from build123d import *

# Parameters (mm, degrees)
F0_R     = 1.55
F1_DEPTH = 3
F3_DEPTH = 3
F4_R     = 1.25
F5_DEPTH = 3
F6_SIZE  = 0.5


with BuildPart() as f1:
    # F0 (on Top) → F1 (new body)
    with BuildSketch(Plane.XY):
        with BuildLine():
            Line((19, 25), (-51, 25))
            ThreePointArc((-51, 25), (-51.707107, 24.707107), (-52, 24))
            Line((-52, 24), (-52, 19.163332))
            Line((-52, 19.163332), (-52, 5.836668))
            Line((-52, 5.836668), (-52, 1))
            ThreePointArc((-52, 1), (-51.707107, 0.292893), (-51, 0))
            Line((-51, 0), (19, 0))
            ThreePointArc((19, 0), (19.707107, 0.292893), (20, 1))
            Line((20, 1), (20, 5.836668))
            Line((20, 5.836668), (20, 19.163332))
            Line((20, 19.163332), (20, 24))
            ThreePointArc((20, 24), (19.707107, 24.707107), (19, 25))
        make_face()
        with BuildLine():
            Line((-52, 5.836668), (-52, 19.163332))
            ThreePointArc((-52, 19.163332), (-52.97063, 17.448574), (-54.940397, 17.398211))
            ThreePointArc((-54.940397, 17.398211), (-63.1, 12.5), (-54.940397, 7.601789))
            ThreePointArc((-54.940397, 7.601789), (-52.97063, 7.551426), (-52, 5.836668))
        make_face()
        with Locations((-57.55, 12.5)):
            Circle(F0_R, mode=Mode.SUBTRACT)
        with BuildLine():
            ThreePointArc((22.940397, 17.398211), (20.97063, 17.448574), (20, 19.163332))
            Line((20, 19.163332), (20, 5.836668))
            ThreePointArc((20, 5.836668), (20.97063, 7.551426), (22.940397, 7.601789))
            ThreePointArc((22.940397, 7.601789), (31.1, 12.5), (22.940397, 17.398211))
        make_face()
        with Locations((25.55, 12.5)):
            Circle(F0_R, mode=Mode.SUBTRACT)
    extrude(amount=F1_DEPTH)

    # F2 (on face) → F3 (join, through all)
    with BuildSketch(Plane.XY.offset(3)):
        with BuildLine():
            Line((-4.25, 25), (-3.75, 25))
            Line((-3.75, 25), (-1.25, 25))
            Line((-1.25, 25), (-0.75, 25))
            ThreePointArc((-0.75, 25), (-1.103553, 25.146447), (-1.25, 25.5))
            Line((-1.25, 25.5), (-1.25, 27.75))
            ThreePointArc((-1.25, 27.75), (-2.5, 29), (-3.75, 27.75))
            Line((-3.75, 27.75), (-3.75, 25.5))
            ThreePointArc((-3.75, 25.5), (-3.896447, 25.146447), (-4.25, 25))
        make_face()
    extrude(amount=-F3_DEPTH)

    # F4 (on face) → F5 (join)
    with BuildSketch(Plane(origin=(0, 0, 0), x_dir=(1, 0, 0), z_dir=(0, 0, -1))):
        with Locations((-2.5, -27.75)):
            Circle(F4_R)
    extrude(amount=F5_DEPTH)

    # F6
    f6_edges = [f1.edges().sort_by_distance(p)[0] for p in [
        (-3.75, 27.75, -3),
    ]]
    chamfer(f6_edges, length=F6_SIZE)


solid = f1.part
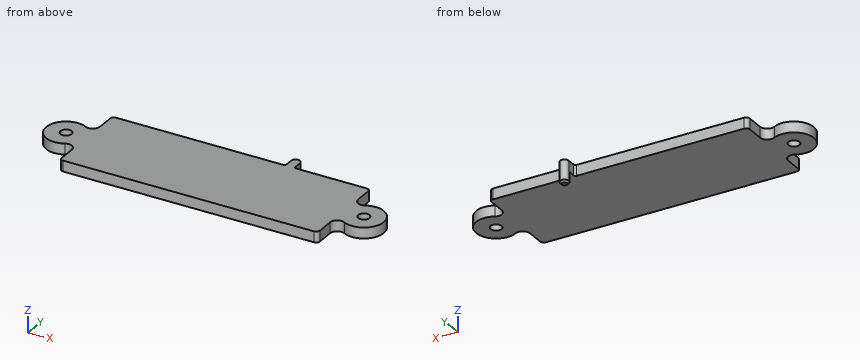
Can you work these out from the model? Positions are in its coordinate system, mm. Coordinates: 2 decimals unless noted, no trailing zeros. Write each loop counter-clockwise with the first axis right and the second up, starting at its lowest first coordinate (ties: lowest second). Pieces come first, ordered by that corner, then holes. Notation, with made-up numbers: M -23,21.25 L 30,21.25 A30 ccw 30,48.25 Z; hole C 18,36 d7. An arc over 180 degrees is marked long. Use one line per item in the form item = value.
Q1. If we section it at B-B (x = -57.55): Write out the boundary of the cut face in (y, z), then the cut area to 3 significant figures.
Model answer:
outline = M 6.95,0 L 10.95,0 L 10.95,3 L 6.95,3 Z; M 14.05,0 L 18.05,0 L 18.05,3 L 14.05,3 Z
area = 24.0 mm^2
Q2. If we section it at A-A (y = 12.5): Write out the boundary of the cut face in (x, z).
Model answer:
outline = M -63.1,0 L -59.1,0 L -59.1,3 L -63.1,3 Z; M -56,0 L 24,0 L 24,3 L -56,3 Z; M 27.1,0 L 31.1,0 L 31.1,3 L 27.1,3 Z
Q3. For P1, Ø2, axis at x = -35, y = 7, coming from the -Z side; P2, Ø2.5, axis at x = 9.5, z = 2, coming from the +Y side; P3, Ø2.5, axis at y = 26.5, z = 1.5, coming from the +X side, each with a flat end and sliding along its axis, tell me the tip position at first contact or that it passes through.
Model answer:
P1 = 0
P2 = 25
P3 = -1.18
Q4. If we section it at D-D (x = 5): Write out the boundary of the cut face in (y, z), then the cut area to 3 significant figures.
Model answer:
outline = M 0,0 L 25,0 L 25,3 L 0,3 Z
area = 75.0 mm^2
Q5. If we section it at C-C (z = 0.95): Write out the boundary of the cut face in (x, y), then the cut area to 3 significant figures.
Model answer:
outline = M -54.94,7.6 A2 cw -52,5.84 L -52,1 A1 ccw -51,0 L 19,0 A1 ccw 20,1 L 20,5.84 A2 cw 22.94,7.6 A5.55 ccw long 22.94,17.4 A2 cw 20,19.16 L 20,24 A1 ccw 19,25 L -0.75,25 A0.5 cw -1.25,25.5 L -1.25,27.75 A1.25 ccw -3.75,27.75 L -3.75,25.5 A0.5 cw -4.25,25 L -51,25 A1 ccw -52,24 L -52,19.16 A2 cw -54.94,17.4 A5.55 ccw long Z; hole C -57.55,12.5 d3.1; hole C 25.55,12.5 d3.1
area = 2,000 mm^2
Q6. I need wall thicknesses on line 1 along Y through (x, z) = (-57.55, 1); line 2 along Y through (x, z) = (-43, 2.65); line 3 along X through (y, z) = (2.5, 0.05). Which ranges of each line are inside material? Lowest first, please. Write a range as from..to.
Model answer:
line_1 = 6.95..10.95, 14.05..18.05
line_2 = 0..25
line_3 = -52..20
